Can you work these out from the model? Positions are in its coordinate system, mm. Round coordinates to 2 decimals unless told otherwise and drop trailing zeros. Loops run counter-clockwise (first coordinate to the right, second up) from the corner with the lowest first, then second, coordinate; pieces in that order, holes last. Notation, with made-up numbers: (84, 19.25) -> (92, 19.25) arc R4 cw to (92, 24.25) -> close; hole circle Ø2 at (13.25, -33.5). An arc over 180 degrees is marked (long way). Use a Markdown table: item, result.
from build123d import *

# Parameters (mm, degrees)
F0_W     = 20
F0_H     = 200
F1_DEPTH = 2
F2_R     = 4
F3_DEPTH = 12.5
F4_R     = 6
F4_R_2   = 4
F5_DEPTH = 2
F8_DEPTH = 25


with BuildPart() as f1:
    # F0 (on Top) → F1 (new body)
    with BuildSketch(Plane.XY):
        Rectangle(F0_W, F0_H)
        with BuildLine():
            Line((-10, 100), (10, 100))
            ThreePointArc((10, 100), (0, 110), (-10, 100))
        make_face()
        with BuildLine():
            ThreePointArc((-10, -100), (0, -110), (10, -100))
            Line((10, -100), (-10, -100))
        make_face()
    extrude(amount=F1_DEPTH)

    # F2 (on Top) → F3 (cut, symmetric)
    with BuildSketch(Plane.XY):
        with Locations((0, 100)):
            Circle(F2_R)
        Circle(F2_R)
        with Locations((0, -100)):
            Circle(F2_R)
    extrude(amount=F3_DEPTH, both=True, mode=Mode.SUBTRACT)

    # F7 (on face) → F8 (cut)
    with BuildSketch(Plane.XY.offset(2)):
        with BuildLine():
            ThreePointArc((10, 0), (0, -10), (-10, 0))
            Line((-10, 0), (-10, -100))
            ThreePointArc((-10, -100), (0, -110), (10, -100))
            Line((10, -100), (10, 0))
        make_face()
    extrude(amount=-F8_DEPTH, mode=Mode.SUBTRACT)


with BuildPart() as f5:
    # F4 (on face) → F5 (new body)
    with BuildSketch(Plane.XY.offset(2)):
        Circle(F4_R)
        Circle(F4_R_2, mode=Mode.SUBTRACT)
    extrude(amount=F5_DEPTH)


solid = f1.part
1. I want a section at D-D (x = -5.25). Please give me the cut outline in (y, z), plus the area to 3 significant figures.
Answer sheet:
| item | result |
|---|---|
| outline | (-8.51, 0) -> (108.51, 0) -> (108.51, 2) -> (-8.51, 2) -> close |
| area | 234 mm² |
2. If we mould it in two halves opening along Y, with no side actions, what happens to faces 1 (the cylindrical face through (-0.867, -3.905, 0.986)), 2 (the flat face through (-10, 49, 1)), 3 (the cylindrical face through (0, -10, 1))? For each: +Y half, -Y half, draft (parallel to the pull), parting line (faces both ways), or undercut.
Answer sheet:
| item | result |
|---|---|
| face 1 | undercut |
| face 2 | draft |
| face 3 | -Y half |
3. I want a section at C-C (x = 7). Please give me the cut outline in (y, z).
Answer sheet:
| item | result |
|---|---|
| outline | (-7.14, 0) -> (107.14, 0) -> (107.14, 2) -> (-7.14, 2) -> close |
4. I want a section at A-A (x = 0). Please give me the cut outline in (y, z), plus the area to 3 significant figures.
Answer sheet:
| item | result |
|---|---|
| outline | (-10, 0) -> (-4, 0) -> (-4, 2) -> (-10, 2) -> close; (4, 0) -> (96, 0) -> (96, 2) -> (4, 2) -> close; (104, 0) -> (110, 0) -> (110, 2) -> (104, 2) -> close |
| area | 208 mm² |
5. Will this pin go through, and if not, where does the flat tip stop? pin 1 Ø9 at (x, y) = (0, 100) entering from +Z.
Answer sheet:
| item | result |
|---|---|
| pin 1 | stops at z = 2 |
6. I need wall thicknesses on line 1 (Y direction, x = 0, z = 1.65); line 2 (X direction, y = 0, z = 1.2); line 3 (Y direction, x = 2.5, z = 1.3). Which ranges of each line are inside material? Lowest first, please.
Answer sheet:
| item | result |
|---|---|
| line 1 | y = -10 to -4, 4 to 96, 104 to 110 |
| line 2 | x = -10 to -4, 4 to 10 |
| line 3 | y = -9.68 to -3.12, 3.12 to 96.88, 103.12 to 109.68 |
7. I want a section at B-B (z = 1.5). Please give me the cut outline in (x, y), plus the area to 3 significant figures.
Answer sheet:
| item | result |
|---|---|
| outline | (-10, 0) arc R10 ccw to (10, 0) -> (10, 100) arc R10 ccw to (-10, 100) -> close; hole circle Ø8 at (0, 0); hole circle Ø8 at (0, 100) |
| area | 2,210 mm² |
